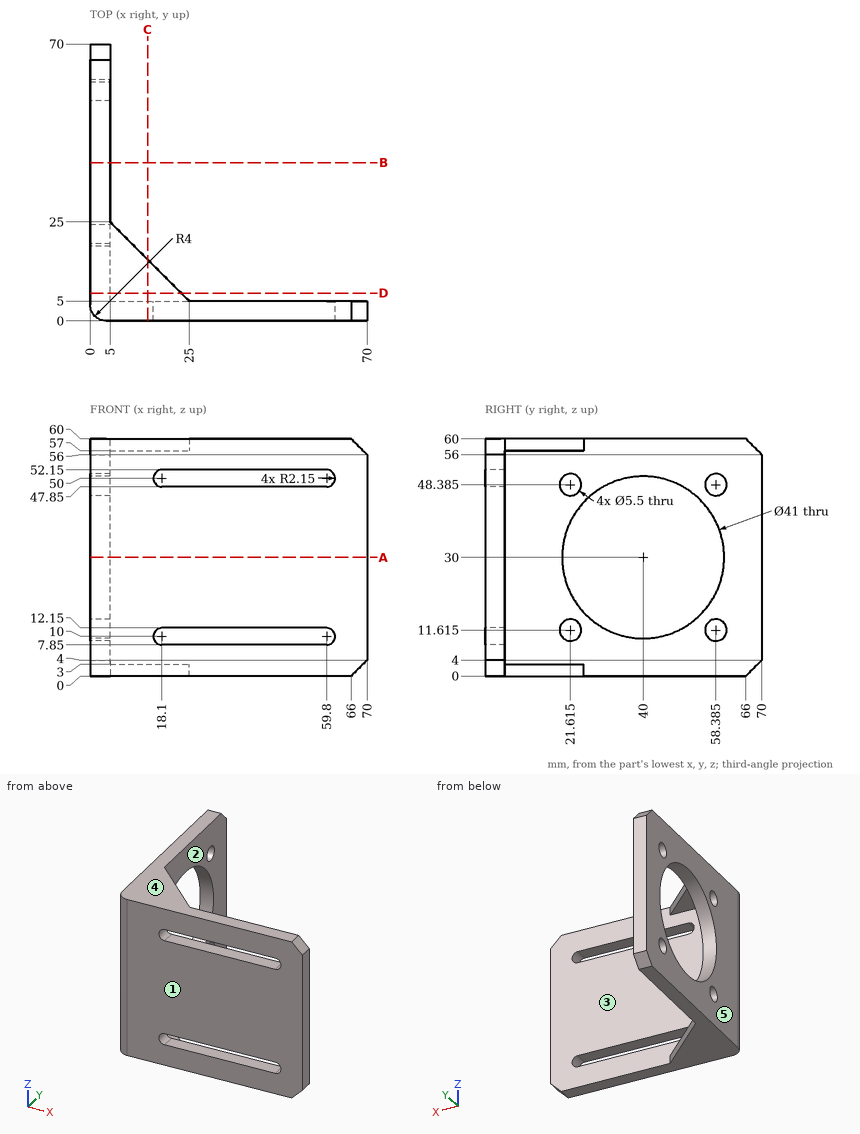
Answer from the drawing. Dimensions are ordinates in mm from the lowest x, y and z of the part. A direction names the side the tool comes from. Coordinates: 2 decimals unless noted, no trailing zeros. Order: outer loops, then holes, each group sorted by start corner. A loop starts at its lowest first (then second) coordinate and runs counter-clockwise, first axis right, second up. Notation, with made-up numbers: (14, 28.25) - (62, 28.25) arc R14 ccw to (62, 49.25) - close; hole circle Ø6 at (57, 44). An arc over 180 degrees is marked (long way). Put each result on its own line as item: value. Start each with the question number.
1) For a pull along Z with two mould halves and no side action, classify the marked faces 3, 4 and 5 as released by +Z, released by -Z, zero draft, split by the parting line, or undercut.
2) Find section A-A (z = 30). Give the vertices of the cut face in (x, y).
3) Flat-ended cylindrical pins translate along their axes: pin 1 (1 mm diameter, centred on x = 55, z = 29, fed in from +Y); pin 2 (6 mm diameter, centred on y = 31, z = 10, fed in from +X). Find the tip coordinate at first contact, or state that the pin passes through.
4) Find section D-D (y = 7). Give the vertices of the cut face in (x, z).
5) For the marked faces 1 and 2, determine the directions among +Z, -Z, +X, -X, +Y, -Y from which every point of the face is accessible in a straight line to the end or side of a thin tool.
6) Find section B-B (y = 40). Give the vertices of the cut face in (x, z), plus the area to 3 significant figures.
7) Find the intervals of material crossed by line 1 (Z direction, x = 1.1, y = 40); line 2 (Y direction, x = 55.5, z = 52.5), in increasing order. Write a range as from..to.
8) Find section C-C (x = 14.5). Give the vertices of the cut face in (y, z).
Results list:
1. face 3: undercut
1. face 4: released by +Z
1. face 5: zero draft
2. outline: (0, 4) arc R4 ccw to (4, 0) - (70, 0) - (70, 5) - (5, 5) - (5, 19.5) - (0, 19.5) - close; (0, 60.5) - (5, 60.5) - (5, 70) - (0, 70) - close
3. pin 1: stops at y = 5
3. pin 2: stops at x = 5
4. outline: (0, 0) - (23, 0) - (23, 3) - (5, 3) - (5, 57) - (23, 57) - (23, 60) - (0, 60) - close
5. face 1: +Z, -Z, +X, -X, -Y
5. face 2: +X, +Y
6. outline: (0, 0) - (5, 0) - (5, 9.5) - (0, 9.5) - close; (0, 50.5) - (5, 50.5) - (5, 60) - (0, 60) - close
6. area: 95.0 mm^2
7. line 1: z = 0..9.5, 50.5..60
7. line 2: y = 0..5
8. outline: (0, 0) - (15.5, 0) - (15.5, 3) - (5, 3) - (5, 57) - (15.5, 57) - (15.5, 60) - (0, 60) - close
